Source: three-view drawing plus pictorial views. Frame: mm from the lowest corner of the part. Coordinates: 2 decimals unless noted, no trailing zeros. Order: outer loops, then holes, each group sorted by start corner. A loop starts at its lowest first (then second) coordinate and runs counter-clockwise, first axis right, second up. Notation, with made-up numbers: (33, 84.5) - (72, 84.5) arc R26 cw to (72, 123.5) - close; hole circle Ø4 at (24, -34). An arc over 180 degrees is marked (long way). One line per question, with ' | ' between items.
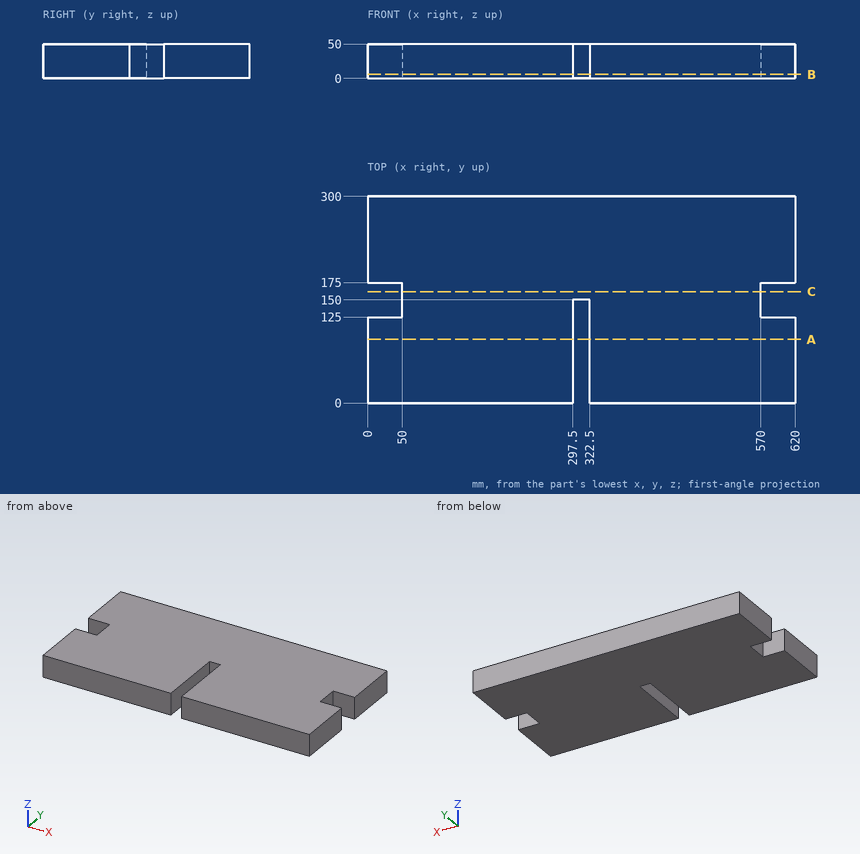
Item 1: Section B-B on z = 6. Return the cut outline in (x, y).
Data:
outline: (0, 0) - (297.5, 0) - (297.5, 150) - (322.5, 150) - (322.5, 0) - (620, 0) - (620, 125) - (570, 125) - (570, 175) - (620, 175) - (620, 300) - (0, 300) - (0, 175) - (50, 175) - (50, 125) - (0, 125) - close
Item 2: Section C-C on y = 162. Return the cut outline in (x, z).
Data:
outline: (50, 0) - (570, 0) - (570, 50) - (50, 50) - close
Item 3: Section A-A on y = 92.5. Return the cut outline in (x, z), and give its area (4 significant figures).
Data:
outline: (0, 0) - (297.5, 0) - (297.5, 50) - (0, 50) - close; (322.5, 0) - (620, 0) - (620, 50) - (322.5, 50) - close | area: 29,750 mm^2
Item 4: Contact query for a flat-ended pin moving along its axis: P1, Ø12.5, axis at x = 311, z = 33.5, coming from the -Y side. Output: stop coordinate, or through.
Data:
P1: y = 150
Item 5: Ray query, line 1 (X direction, y = 46, z = 21); line 2 (Y direction, x = 43.5, z = 32.5); line 3 (X direction, y = 139.5, z = 44.5). Return the intervals inside material, ascending.
Data:
line 1: 0 to 297.5, 322.5 to 620 | line 2: 0 to 125, 175 to 300 | line 3: 50 to 297.5, 322.5 to 570
